from build123d import *

# Parameters (mm, degrees)
SKETCH1_R                                   = 3
QUADRADO_PF20_01_PERFIL_2020_B_SICO_1_DEPTH = 315.6


with BuildPart() as part:
    # Sketch1 → Quadrado PF20-01 - PERFIL 2020 BÁSICO(1) (new body)
    with BuildSketch(Plane.YZ):
        with BuildLine():
            Line((8.187867966, -7.26862915), (4.439339828, -3.520101013))
            ThreePointArc((4.439339828, -3.520101013), (4.114180701, -3.033465989), (4, -2.459440841))
            Line((4, -2.459440841), (4, 2.459440841))
            ThreePointArc((4, 2.459440841), (4.114180701, 3.033465989), (4.439339828, 3.520101013))
            Line((4.439339828, 3.520101013), (8.187867966, 7.26862915))
            ThreePointArc((8.187867966, 7.26862915), (8.51480503, 7.333660975), (8.7, 7.056497116))
            Line((8.7, 7.056497116), (8.7, 4))
            Line((8.7, 4), (10, 4))
            Line((10, 4), (10, 9.5))
            ThreePointArc((10, 9.5), (9.853553391, 9.853553391), (9.5, 10))
            Line((9.5, 10), (4, 10))
            Line((4, 10), (4, 8.7))
            Line((4, 8.7), (7.056497116, 8.7))
            ThreePointArc((7.056497116, 8.7), (7.333660975, 8.51480503), (7.26862915, 8.187867966))
            Line((7.26862915, 8.187867966), (3.520101013, 4.439339828))
            ThreePointArc((3.520101013, 4.439339828), (3.033465989, 4.114180701), (2.459440841, 4))
            Line((2.459440841, 4), (-2.459440841, 4))
            ThreePointArc((-2.459440841, 4), (-3.033465989, 4.114180701), (-3.520101013, 4.439339828))
            Line((-3.520101013, 4.439339828), (-7.26862915, 8.187867966))
            ThreePointArc((-7.26862915, 8.187867966), (-7.333660975, 8.51480503), (-7.056497116, 8.7))
            Line((-7.056497116, 8.7), (-4, 8.7))
            Line((-4, 8.7), (-4, 10))
            Line((-4, 10), (-9.5, 10))
            ThreePointArc((-9.5, 10), (-9.853553391, 9.853553391), (-10, 9.5))
            Line((-10, 9.5), (-10, 4))
            Line((-10, 4), (-8.7, 4))
            Line((-8.7, 4), (-8.7, 7.056497116))
            ThreePointArc((-8.7, 7.056497116), (-8.51480503, 7.333660975), (-8.187867966, 7.26862915))
            Line((-8.187867966, 7.26862915), (-4.439339828, 3.520101013))
            ThreePointArc((-4.439339828, 3.520101013), (-4.114180701, 3.033465989), (-4, 2.459440841))
            Line((-4, 2.459440841), (-4, -2.459440841))
            ThreePointArc((-4, -2.459440841), (-4.114180701, -3.033465989), (-4.439339828, -3.520101013))
            Line((-4.439339828, -3.520101013), (-8.187867966, -7.26862915))
            ThreePointArc((-8.187867966, -7.26862915), (-8.51480503, -7.333660975), (-8.7, -7.056497116))
            Line((-8.7, -7.056497116), (-8.7, -4))
            Line((-8.7, -4), (-10, -4))
            Line((-10, -4), (-10, -9.5))
            ThreePointArc((-10, -9.5), (-9.853553391, -9.853553391), (-9.5, -10))
            Line((-9.5, -10), (-4, -10))
            Line((-4, -10), (-4, -8.7))
            Line((-4, -8.7), (-7.056497116, -8.7))
            ThreePointArc((-7.056497116, -8.7), (-7.333660975, -8.51480503), (-7.26862915, -8.187867966))
            Line((-7.26862915, -8.187867966), (-3.520101013, -4.439339828))
            ThreePointArc((-3.520101013, -4.439339828), (-3.033465989, -4.114180701), (-2.459440841, -4))
            Line((-2.459440841, -4), (2.459440841, -4))
            ThreePointArc((2.459440841, -4), (3.033465989, -4.114180701), (3.520101013, -4.439339828))
            Line((3.520101013, -4.439339828), (7.26862915, -8.187867966))
            ThreePointArc((7.26862915, -8.187867966), (7.333660975, -8.51480503), (7.056497116, -8.7))
            Line((7.056497116, -8.7), (4, -8.7))
            Line((4, -8.7), (4, -10))
            Line((4, -10), (9.5, -10))
            ThreePointArc((9.5, -10), (9.853553391, -9.853553391), (10, -9.5))
            Line((10, -9.5), (10, -4))
            Line((10, -4), (8.7, -4))
            Line((8.7, -4), (8.7, -7.056497116))
            ThreePointArc((8.7, -7.056497116), (8.51480503, -7.333660975), (8.187867966, -7.26862915))
        make_face()
        Circle(SKETCH1_R, mode=Mode.SUBTRACT)
    extrude(amount=QUADRADO_PF20_01_PERFIL_2020_B_SICO_1_DEPTH)


solid = part.part
Could you check a few things on this model? Use its own coordinates, in mm. A direction names the side the tool comes from. Coordinates: 2 decimals unless noted, no trailing zeros.
1. We'd pull the mould along Z, two halves only. Please class faces 1 (the face through (156, -4, 0)), 2 (the face through (156, -7, -10)), 3 (the face through (156, 4, 0)), 4 (the face through (156, 10, -7)): released by +Z, released by -Z, zero draft, split by the parting line, or undercut.
2. For faces 5 (the face through (156, 0, -4)), 6 (the face through (156, 0, 4)), 7 (the face through (156, -3, 0)), which set-ups out of +Z, -Z, +X, -X, +Y, -Y let a thin tool reach every point of the face, with its end or its side?
3. For P1, Ø4, axis at x = 165.5, y = 0, coming from the -Z side; P2, Ø1.5, axis at x = 102.5, y = 1, coming from the +Z side; P3, Ø2.5, axis at x = 226.5, z = 0.5, coming from the +Y side, each with a flat end and sliding along its axis, tell me the tip position at first contact or that it passes through.
4. I need wall thicknesses on L1, parallel to Z at x = 247, y = -1.75; L2, parallel to Z at x = 203, y = 0. Which ranges of each line are inside material? Lowest first, please.
Computed values:
1. face 1: undercut
1. face 2: released by -Z
1. face 3: undercut
1. face 4: zero draft
2. face 5: -Z, +X, -X
2. face 6: +Z, +X, -X
2. face 7: +X, -X
3. P1: stops at z = -4
3. P2: stops at z = 4
3. P3: stops at y = 4
4. L1: z = -4 to -2.44, 2.44 to 4
4. L2: z = -4 to -3, 3 to 4
